CAD build for the part. Positions are in the model's coordinates, mm. Face numbers are marked on the shaded views. A direction names the side the tool comes from. Round coordinates to 2 decimals unless told otherwise and drop trailing zeros. Loops run counter-clockwise (first coordinate to the right, second up) from the corner with the lowest first, then second, coordinate; pieces in that order, holes last. Notation, with made-up numbers: M -34.75,-32 L -22.75,-32 A14 cw -22.75,-24 Z; hole C -4,-37.5 d5. An arc over 180 degrees is marked long. One line per item, written item: value. Start each with the question number.
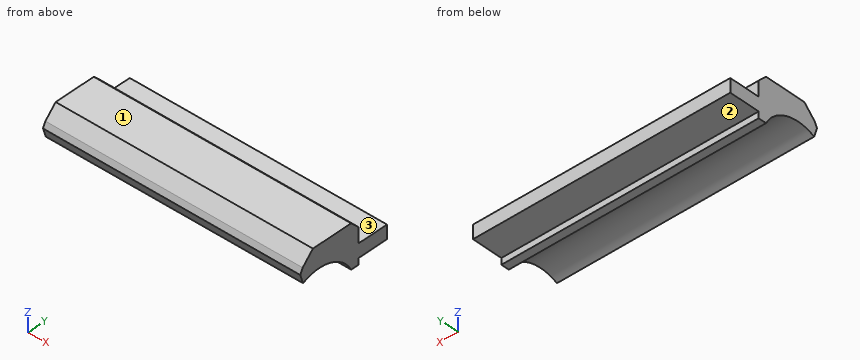
from build123d import *

# Parameters (mm, degrees)
BOSS_EXTRUDE2_DEPTH = 10


with BuildPart() as part:
    # Sketch1 → Boss-Extrude2 (new body)
    with BuildSketch(Plane(origin=(0, 0, 0), x_dir=(0, 0, -1), z_dir=(1, 0, 0))):
        with BuildLine():
            Line((0.181484262, 0.201549296), (-0.348515738, 0.201549296))
            Line((-0.348515738, 0.201549296), (-0.348515738, -0.987434189))
            Line((-0.348515738, -0.987434189), (-0.933817853, -0.987434189))
            Line((-0.933817853, -0.987434189), (-1.25063724, -1.304253576))
            Line((-1.25063724, -1.304253576), (-1.25063724, -2.902375908))
            Line((-1.25063724, -2.902375908), (-0.806436057, -3.331336004))
            Line((-0.806436057, -3.331336004), (-0.598754104, -3.432629261))
            Line((-0.598754104, -3.432629261), (-0.234865404, -3.314394655))
            ThreePointArc((-0.234865404, -3.314394655), (-0.321657185, -2.169629757), (0.42644278, -1.298787678))
            Line((0.42644278, -1.298787678), (0.42644278, -0.987434189))
            Line((0.42644278, -0.987434189), (0.181484262, -0.987434189))
            Line((0.181484262, -0.987434189), (0.181484262, 0.201549296))
        make_face()
    extrude(amount=BOSS_EXTRUDE2_DEPTH)


solid = part.part
(1) Slice it at C-C, the plane z = -0.3. List the corners of the cut face in (x, y), and give its area (3 significant figures).
(2) Slice it at A-A, the plane x = 4.5. List the corners of the cut face in (y, z), and give its area (3 significant figures).
(3) Slice it at B-B, the plane y = -0.9. List the corners of the cut face in (x, z), and give its area (3 significant figures).
(4) Flat gauge pins, fed straight in: P1, Ø1.3, axis at x = 6, y = -0.5, coming from the +Z side; P2, Ø0.6, axis at x = 4.5, y = -0.5, coming from the -Z side. Where does each tip first touch, or does it go through?
(5) Which spindle directions (+Z, -Z, +X, -X, +Y, -Y) get a long thin tool onto all of the face, cutting with end or side? Do the marked faces 1, 2 and 3. Say none if no direction does.
(6) Probe L1, parallel to Z at x = 7.25, y = -0.95; L2, parallel to Z at x = 2.75, y = -2.7; L3, parallel to Y at x = 5.5, z = 0.7. List the from-to ranges inside material, lowest first.
Check result:
1. outline: M 0,-1.37 L 10,-1.37 L 10,-0.99 L 0,-0.99 Z
1. area: 3.83 mm^2
2. outline: M -3.43,0.6 L -3.31,0.23 A1.5 cw -1.3,-0.43 L -0.99,-0.43 L -0.99,-0.18 L 0.2,-0.18 L 0.2,0.35 L -0.99,0.35 L -0.99,0.93 L -1.3,1.25 L -2.9,1.25 L -3.33,0.81 Z
2. area: 3.12 mm^2
3. outline: M 0,-0.18 L 10,-0.18 L 10,0.35 L 0,0.35 Z
3. area: 5.30 mm^2
4. P1: stops at z = 1.1
4. P2: stops at z = -0.18
5. face 1: +Z, +X, -X, +Y, -Y
5. face 2: -Z, +X, -X, +Y
5. face 3: +Z, +X, -X, +Y
6. L1: z = -0.18 to 0.35
6. L2: z = 0.4 to 1.25
6. L3: y = -3.38 to -0.99
